Check sheet for the drawn part. Datum: minimum x, y, z corner. Units: mm. Coordinates: 2 decimals unless noted, no trailing zeros. Write each loop counter-clockwise with the first axis right and the second up, starting at its lowest first coordinate (ties: lowest second). Pieces come first, ordered by that corner, then holes. Notation, with made-up numbers: (72, -32) -> (131, -32) arc R27 cw to (131, -11) -> close; hole circle Ø9 at (36, -30). An arc over 180 degrees is marked (long way). One line per question, with ' | ' between items.
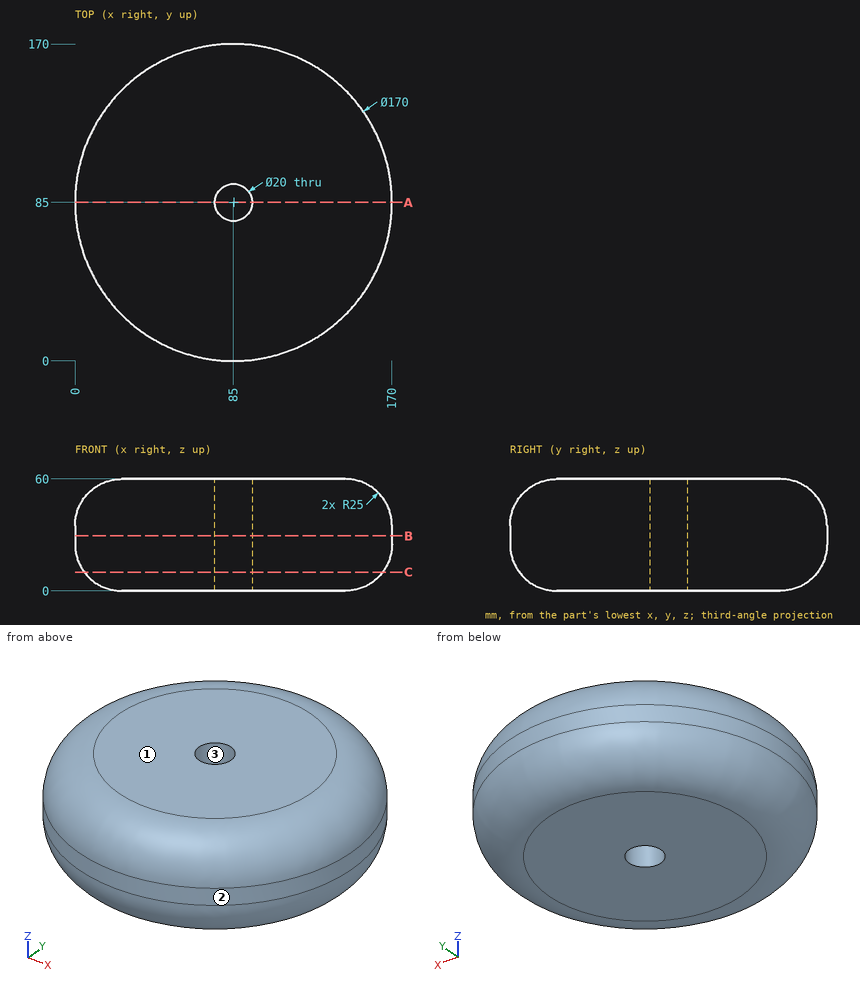
1. Mould release check, pull along Y, two halves, no side actions. Record for the marked faces 1, 2 and 3: released by +Y, released by -Y, zero draft, split by the parting line, or undercut.
Worked answers:
face 1: zero draft | face 2: split by the parting line | face 3: undercut
2. Cross-section at A-A on y = 85. Record the boundary of the cut face in (x, z), and give its area (3 significant figures).
Worked answers:
outline: (0, 25) arc R25 ccw to (25, 0) -> (75, 0) -> (75, 60) -> (25, 60) arc R25 ccw to (0, 35) -> close; (95, 0) -> (145, 0) arc R25 ccw to (170, 25) -> (170, 35) arc R25 ccw to (145, 60) -> (95, 60) -> close | area: 8,460 mm²
3. Go/stop test with flat-tipped pins: P1, Ø8, axis at x = 49.5, z = 30, coming from the +Y side; P2, Ø1.5, axis at y = 118, z = 13, coming from the -X side; P3, Ø1, axis at x = 48, z = 48, coming from the +Y side; P4, Ø18, axis at x = 85, y = 85, coming from the +Z side. Record where each tip stops, or that it passes through.
Worked answers:
P1: y = 163.95 | P2: x = 9.47 | P3: y = 157.87 | P4: through
4. Cross-section at B-B on z = 29.5. Record the boundary of the cut face in (x, y), and give its area (3 significant figures).
Worked answers:
outline: circle Ø170 at (85, 85); hole circle Ø20 at (85, 85) | area: 22,400 mm²
5. Cross-section at C-C on z = 10. Record the boundary of the cut face in (x, y).
Worked answers:
outline: circle Ø160 at (85, 85); hole circle Ø20 at (85, 85)
6. Material ranges on line 1 (Y direction, x = 85, z = 32); line 2 (Y direction, x = 85, z = 38); line 3 (Z direction, x = 80.5, y = 161), recorded low to high. Write a range as from..to.
Worked answers:
line 1: 0..75, 95..170 | line 2: 0.18..75, 95..169.82 | line 3: 5.9..54.1
